Input: dimensioned drawing with shaded views. Units: mm. Origin: part minimum x, y, z. Give positions to 0.01 mm unless a question says otherwise; leave off trailing zeros. Order: outer loops, then holes, each group sorted by start corner. A loop starts at its lowest first (then second) coordinate and runs counter-clockwise, first axis right, second up.
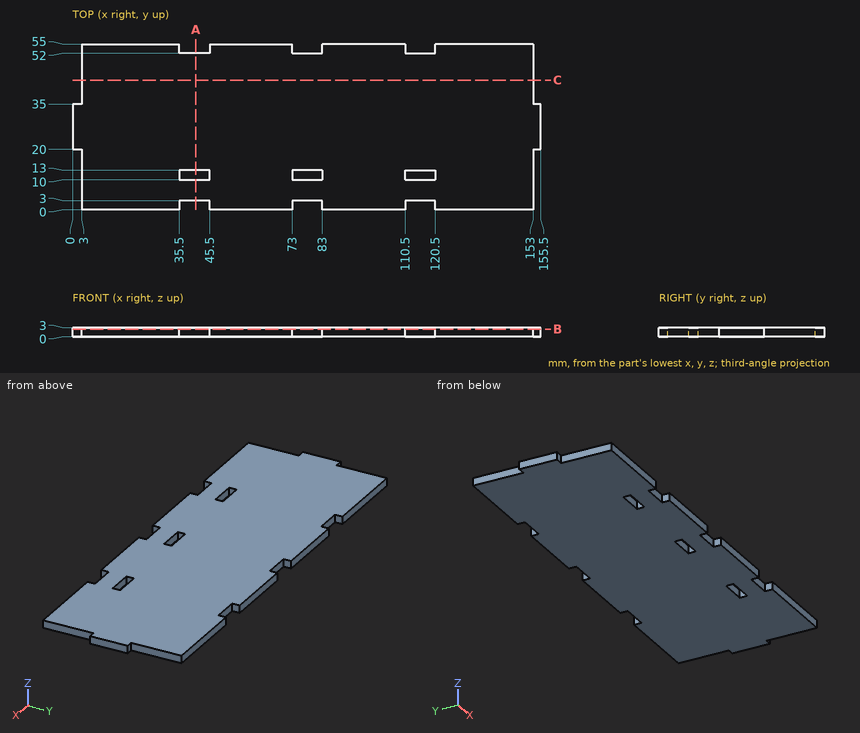
1) Section query A-A, the plane x = 41. Return the cut outline in (y, z), and give its area (3 significant figures).
Report:
outline: (3, 0) - (10, 0) - (10, 3) - (3, 3) - close; (13, 0) - (52, 0) - (52, 3) - (13, 3) - close
area: 138 mm2
2) Section query B-B, the plane z = 2.55. Count the separate pieces of the cut face and the enclosed holes in it, and give its area (3 significant figures).
Report:
separate pieces: 1
enclosed holes: 3
area: 8,060 mm2
3) Material intervals for L1, parallel to Y at x = 81.5, z = 0.6; L2, parallel to X at y = 45, z = 1.65, sorted ascending.
Report:
L1: y = 3 to 10, 13 to 52
L2: x = 3 to 153
4) Pin query (flat end, axial travel): pin 1 (0.9 mm diameter, centred on y = 12, z = 1.5, fed in from -X); pin 2 (0.9 mm diameter, centred on y = 43, z = 1.5, fed in from +X); pin 3 (1.5 mm diameter, centred on x = 117, z = 1, fed in from +Y). Return the tip coordinate at first contact, or that it passes through.
Report:
pin 1: stops at x = 3
pin 2: stops at x = 153
pin 3: stops at y = 52
5) Section query C-C, the plane y = 43. Return the cut outline in (x, z), and give its area (3 significant figures).
Report:
outline: (3, 0) - (153, 0) - (153, 3) - (3, 3) - close
area: 450 mm2
